from build123d import *

# Parameters (mm, degrees)
F1_DEPTH = 2


with BuildPart() as f1:
    # F0 (on Top) → F1 (new body)
    with BuildSketch(Plane.XY):
        with BuildLine():
            Line((-22.272078, 35), (-55.485458, 68.21338))
            ThreePointArc((-55.485458, 68.21338), (-70.717514, 70.717514), (-68.21338, 55.485458))
            Line((-68.21338, 55.485458), (-22.272078, 9.544156))
            Line((-22.272078, 9.544156), (-22.272078, 0))
            Line((-22.272078, 0), (-22.272078, -9.544156))
            Line((-22.272078, -9.544156), (-68.21338, -55.485458))
            ThreePointArc((-68.21338, -55.485458), (-70.717514, -70.717514), (-55.485458, -68.21338))
            Line((-55.485458, -68.21338), (-22.272078, -35))
            Line((-22.272078, -35), (22.272078, -35))
            Line((22.272078, -35), (55.485458, -68.21338))
            ThreePointArc((55.485458, -68.21338), (70.717514, -70.717514), (68.21338, -55.485458))
            Line((68.21338, -55.485458), (22.272078, -9.544156))
            Line((22.272078, -9.544156), (22.272078, 0))
            Line((22.272078, 0), (22.272078, 9.544156))
            Line((22.272078, 9.544156), (68.21338, 55.485458))
            ThreePointArc((68.21338, 55.485458), (70.717514, 70.717514), (55.485458, 68.21338))
            Line((55.485458, 68.21338), (22.272078, 35))
            Line((22.272078, 35), (-22.272078, 35))
        make_face()
    extrude(amount=F1_DEPTH)


solid = f1.part
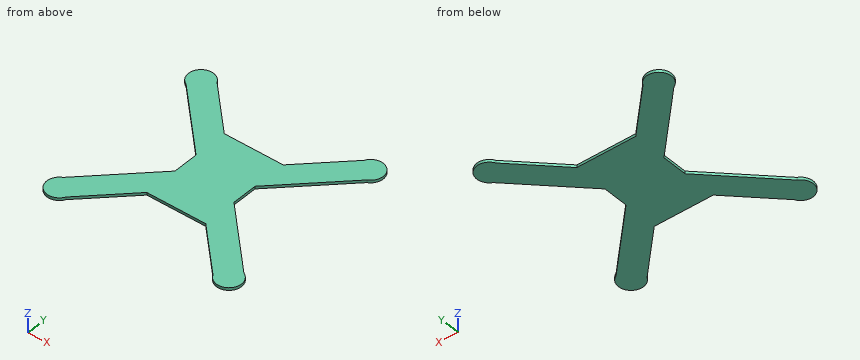
The listing builds one solid part. Answer for the finished solid, in the listing's coordinates (mm). Round coordinates to 2 decimals unless told otherwise and drop trailing zeros. Order: outer loops, then holes, each group sorted by start corner. A loop starts at its lowest first (then second) coordinate and runs counter-clockwise, first axis right, second up. Notation, with made-up numbers: (24.25, -4) - (42.25, -4) arc R7 cw to (42.25, 7) - close; hole circle Ø9 at (49, -4). An arc over 180 degrees is marked (long way). Write item = value, one per line. Start each with the question number.
1) Given pin 1 (12 mm diameter, centred on x = -1.5, y = 38.5, fed in from -Z); pin 2 (0.6 mm diameter, centred on y = 1, z = 0.5, fed in from +X), each flat-ended and moving along its own axis, determine where each tip first touches the part or whether it passes through.
2) Straight lines are drawn through the part: L1, parallel to X at y = -5.5, z = 1.55; L2, parallel to Y at x = -47, z = 1.4; L3, parallel to X at y = 56, z = 1.7. For each, find the intervals that lie inside material, in ascending order.
3) Section D-D, the plane y = 7 is taken. Write down the section's boundary in (x, z), plus the area to 3 significant figures.
4) Section B-B, the plane x = 52.5 is taken. Write down the section's boundary in (y, z), plus the area to 3 significant figures.
5) Section C-C, the plane z = 1.2 is taken. Write down the section's boundary in (x, y).
6) Section A-A, the plane y = 60 is taken. Write down the section's boundary in (x, z).
Results list:
q1.pin_1 = 0
q1.pin_2 = 22.27
q2.L1 = -22.27 to 22.27
q2.L2 = -59.73 to -34.27, 34.27 to 59.73
q2.L3 = -69.12 to -43.27, 43.27 to 69.12
q3.outline = (-22.27, 0) - (22.27, 0) - (22.27, 2) - (-22.27, 2) - close
q3.area = 89.1 mm^2
q4.outline = (-65.23, 0) - (-39.77, 0) - (-39.77, 2) - (-65.23, 2) - close; (39.77, 0) - (65.23, 0) - (65.23, 2) - (39.77, 2) - close
q4.area = 102 mm^2
q5.outline = (-68.21, -55.49) arc R9.5 ccw (long way) to (-55.49, -68.21) - (-22.27, -35) - (22.27, -35) - (55.49, -68.21) arc R9.5 ccw (long way) to (68.21, -55.49) - (22.27, -9.54) - (22.27, 9.54) - (68.21, 55.49) arc R9.5 ccw (long way) to (55.49, 68.21) - (22.27, 35) - (-22.27, 35) - (-55.49, 68.21) arc R9.5 ccw (long way) to (-68.21, 55.49) - (-22.27, 9.54) - (-22.27, -9.54) - close
q6.outline = (-72.62, 0) - (-47.27, 0) - (-47.27, 2) - (-72.62, 2) - close; (47.27, 0) - (72.62, 0) - (72.62, 2) - (47.27, 2) - close
